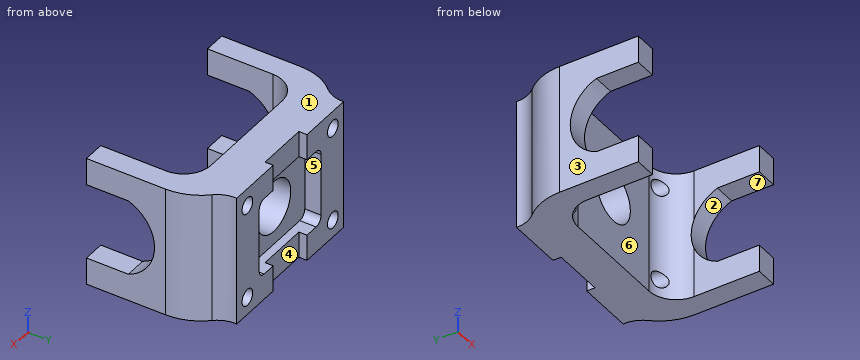
from build123d import *

# Parameters (mm, degrees)
EXTRUDE1_DEPTH          = 60.96
CUT_EXTRUDE1_DEPTH      = 50.893408892
CUT_EXTRUDE1_DEPTH_BACK = 47.626591108
SKETCH5_W               = 44.196
SKETCH5_H               = 36.576
CUT_EXTRUDE3_DEPTH      = 3.81
CUT_EXTRUDE3_DEPTH_BACK = 3.81
FILLET1_R               = 3.556
FILLET2_R               = 3.556
SKETCH6_R               = 12.065
CUT_EXTRUDE4_DEPTH      = 56.88
SKETCH7_R               = 3.81
CUT_EXTRUDE5_DEPTH      = 64.5
LPATTERN1_COUNT         = 2
LPATTERN1_PITCH         = 60.96
LPATTERN1_COUNT_DIR2    = 2
LPATTERN1_PITCH_DIR2    = 44.45


with BuildPart() as part:
    # Sketch1 → Extrude1 (new body)
    with BuildSketch(Plane.XY):
        with BuildLine():
            Line((-4.519970737, -20.32), (7.786788522, -20.32))
            Line((7.786788522, -20.32), (27.033408892, -20.32))
            ThreePointArc((27.033408892, -20.32), (36.013665013, -24.039743879), (39.733408892, -33.02))
            Line((39.733408892, -33.02), (39.733408892, -63.5))
            Line((39.733408892, -63.5), (49.893408892, -63.5))
            Line((49.893408892, -63.5), (49.893408892, -26.67))
            ThreePointArc((49.893408892, -26.67), (48.135622025, -17.385294394), (43.105553917, -9.385670173))
            ThreePointArc((43.105553917, -9.385670173), (40.459641097, -5.037692796), (39.733408892, 0))
            Line((39.733408892, 0), (13.698408892, 0))
            Line((13.698408892, 0), (13.698408892, -3.81))
            Line((13.698408892, -3.81), (-10.431591108, -3.81))
            Line((-10.431591108, -3.81), (-10.431591108, 0))
            Line((-10.431591108, 0), (-36.466591108, 0))
            ThreePointArc((-36.466591108, 0), (-37.192823312, -5.037692796), (-39.838736133, -9.385670173))
            ThreePointArc((-39.838736133, -9.385670173), (-44.868804241, -17.385294394), (-46.626591108, -26.67))
            Line((-46.626591108, -26.67), (-46.626591108, -63.5))
            Line((-46.626591108, -63.5), (-36.466591108, -63.5))
            Line((-36.466591108, -63.5), (-36.466591108, -33.02))
            ThreePointArc((-36.466591108, -33.02), (-32.746847229, -24.039743879), (-23.766591108, -20.32))
            Line((-23.766591108, -20.32), (-4.519970737, -20.32))
        make_face()
    extrude(amount=-EXTRUDE1_DEPTH)

    # Sketch4 → Cut-Extrude1 (cut, two sides)
    with BuildSketch(Plane(origin=(0, 0, 0), x_dir=(0, 0, -1), z_dir=(1, 0, 0))) as cut_extrude1_sk:
        with BuildLine():
            Line((12.7, -233.015235636), (12.7, -63.5))
            Line((12.7, -63.5), (12.7, -43.942))
            ThreePointArc((12.7, -43.942), (30.48, -31.731159305), (48.26, -43.942))
            Line((48.26, -43.942), (48.26, -63.5))
            Line((48.26, -63.5), (48.26, -233.015235636))
            Line((48.26, -233.015235636), (48.26, -572.045706908))
            Line((48.26, -572.045706908), (12.7, -572.045706908))
            Line((12.7, -572.045706908), (12.7, -233.015235636))
        make_face()
    extrude(amount=CUT_EXTRUDE1_DEPTH, mode=Mode.SUBTRACT)
    extrude(cut_extrude1_sk.sketch, amount=-CUT_EXTRUDE1_DEPTH_BACK, mode=Mode.SUBTRACT)

    # Sketch5 → Cut-Extrude3 (cut, two sides)
    with BuildSketch(Plane(origin=(0, -3.81, 0), x_dir=(-1, 0, 0), z_dir=(0, 1, 0))) as cut_extrude3_sk:
        with Locations((-1.633408892, -30.48)):
            Rectangle(SKETCH5_W, SKETCH5_H)
    extrude(amount=CUT_EXTRUDE3_DEPTH, mode=Mode.SUBTRACT)
    extrude(cut_extrude3_sk.sketch, amount=-CUT_EXTRUDE3_DEPTH_BACK, mode=Mode.SUBTRACT)

    # Fillet1
    fillet1_edges = [part.edges().sort_by_distance(p)[0] for p in [
        (23.731408892, -3.81, -12.192),
    ]]
    fillet(fillet1_edges, radius=FILLET1_R)

    # Fillet2
    fillet2_edges = [part.edges().sort_by_distance(p)[0] for p in [
        (23.731408892, -3.81, -48.768),
        (-20.464591108, -3.81, -12.192),
        (-20.464591108, -3.81, -48.768),
    ]]
    fillet(fillet2_edges, radius=FILLET2_R)

    # Sketch6 → Cut-Extrude4 (cut, through all)
    with BuildSketch(Plane(origin=(0, -7.62, 0), x_dir=(-1, 0, 0), z_dir=(0, 1, 0))):
        with Locations((-1.633408892, -30.48)):
            Circle(SKETCH6_R)
    extrude(amount=-CUT_EXTRUDE4_DEPTH, mode=Mode.SUBTRACT)

    # Sketch7 → Cut-Extrude5 (cut, through all)
    with BuildSketch(Plane(origin=(0, 0, 0), x_dir=(-1, 0, 0), z_dir=(0, 1, 0))):
        with Locations((-32.113408892, -8.255)):
            Circle(SKETCH7_R)
    cut_extrude5 = extrude(amount=-CUT_EXTRUDE5_DEPTH, mode=Mode.SUBTRACT)

    # LPattern1: Cut-Extrude5 2 × 2
    with Locations(*[(-i * LPATTERN1_PITCH, 0, -j * LPATTERN1_PITCH_DIR2) for i in range(LPATTERN1_COUNT) for j in range(LPATTERN1_COUNT_DIR2) if (i, j) != (0, 0)]):
        add(cut_extrude5, mode=Mode.SUBTRACT)


solid = part.part
Work out the finished part from the listing and answer in its coordinate system (mm). Face numbers are marked on the shaded views. A direction names the side the tool comes from. Coordinates: 2 decimals unless noted, no trailing zeros. Loops run counter-clockwise (first coordinate to the right, second up) from the corner with the lowest first, then second, coordinate; pieces in that order, holes last. Notation, with made-up numbers: M 5,85 L 31,85 A23 ccw 31,124 Z; hole C 46,51 d8. An arc over 180 degrees is marked long. Answer in a Markdown table with one row per item. Add a question column.
1. Find section C-C, the plane y = -14.5. Write down the section's boundary in (x, z) (3 decimals), then the cut area to 3 significant figures.
2. Find section A-A, the plane x = 11.5. Write down the section's boundary in (y, z).
3. Consider L1, parallel to X at y = -51.5, z = -10; L2, parallel to Y at x = 18.5, z = -37; L3, parallel to X at y = -22, z = -9. Determine where each line is inside the solid, lowest interval first.
4. A tool of negligible diameter and unlimited length cuts with its end or side. For the marked faces 4, 5, 6 and 7, from which of +Z, -Z, +X, -X, +Y, -Y can it reach the whole face along a straight path? Write none if from no direction.
5. Find section B-B, the plane z = -30.48. Write down the section's boundary in (x, y).
6. The mould has two halves that part along Z. Classify the marked faces 1, 2 and 3: pulls with the +Z half, pulls with the -Z half, needs draft (parallel to the pull), parting line crosses it, or undercut.
7. Flat-ended cylindrical pins translate along their axes: P1, Ø1.1, axis at y = -1.5, z = -53.5, coming from the -X side; P2, Ø10, axis at x = 4.5, z = -6.5, coming from the +Y side; P3, Ø2, axis at y = -22.5, z = -48.5, coming from the -X side. Find the tip coordinate at first contact, or state that the pin passes through.
8. Find section D-D, the plane z = -6. Write down the section's boundary in (x, y), then the cut area to 3 significant figures.
Reported:
| question | item | result |
|---|---|---|
| 1 | outline | M -43.521,-60.96 L 46.788,-60.96 L 46.788,0 L -43.521,0 Z; hole C -28.847,-52.705 d7.62; hole C -28.847,-8.255 d7.62; hole C 1.633,-30.48 d24.13; hole C 32.113,-52.705 d7.62; hole C 32.113,-8.255 d7.62 |
| 1 | area | 4,870 mm^2 |
| 2 | outline | M -20.32,-60.96 L -3.81,-60.96 L -3.81,-48.77 L -7.62,-48.77 L -7.62,-37.42 L -20.32,-37.42 Z; M -20.32,-23.54 L -7.62,-23.54 L -7.62,-12.19 L -3.81,-12.19 L -3.81,0 L -20.32,0 Z |
| 3 | L1 | x = -46.63 to -36.47, 39.73 to 49.89 |
| 3 | L2 | y = -20.32 to -7.62 |
| 3 | L3 | x = -46.19 to -32.58, 35.85 to 49.46 |
| 4 | face 4 | +Z, -Z, +Y |
| 4 | face 5 | +Y |
| 4 | face 6 | +Z, -Z, -Y |
| 4 | face 7 | +X, -X, -Y |
| 5 | outline | M -46.63,-31.73 L -36.4,-31.73 A12.7 cw -23.77,-20.32 L -10.43,-20.32 L -10.43,-7.62 L -20.46,-7.62 L -20.46,0 L -36.47,0 A12.7 cw -39.84,-9.39 A25.4 ccw -46.63,-26.67 Z; M 13.7,-20.32 L 27.03,-20.32 A12.7 cw 39.67,-31.73 L 49.89,-31.73 L 49.89,-26.67 A25.4 ccw 43.11,-9.39 A12.7 cw 39.73,0 L 23.73,0 L 23.73,-7.62 L 13.7,-7.62 Z |
| 6 | face 1 | pulls with the +Z half |
| 6 | face 2 | undercut |
| 6 | face 3 | needs draft |
| 7 | P1 | stops at x = -36.51 |
| 7 | P2 | stops at y = -3.81 |
| 7 | P3 | stops at x = -46.43 |
| 8 | outline | M -46.63,-63.5 L -36.47,-63.5 L -36.47,-33.02 A12.7 cw -31.92,-23.28 L -31.92,0 L -36.47,0 A12.7 cw -39.84,-9.39 A25.4 ccw -46.63,-26.67 Z; M -25.78,-20.48 A12.7 cw -23.77,-20.32 L 27.03,-20.32 A12.7 cw 29.04,-20.48 L 29.04,0 L 13.7,0 L 13.7,-3.81 L -10.43,-3.81 L -10.43,0 L -25.78,0 Z; M 35.18,-23.28 A12.7 cw 39.73,-33.02 L 39.73,-63.5 L 49.89,-63.5 L 49.89,-26.67 A25.4 ccw 43.11,-9.39 A12.7 cw 39.73,0 L 35.18,0 Z |
| 8 | area | 2,310 mm^2 |
